```python
from build123d import *

# Parameters (mm, degrees)
SKIZZE2_R = 0.75


with BuildPart() as part:
    # Austragung1: sweep along a path in Skizze1
    with BuildLine(Plane.XY) as austragung1_path:
        Line((0, 0), (0, 15))
        ThreePointArc((0, 15), (-0.782050775, 17.292111995), (-2.802014612, 18.62819841))
        Line((-2.802014612, 18.62819841), (-26.697985388, 24.87180159))
        ThreePointArc((-26.697985388, 24.87180159), (-29.499946504, 28.47996964), (-26.736690272, 32.11786433))
        Line((-26.736690272, 32.11786433), (-4.736690272, 38.11786433))
        ThreePointArc((-4.736690272, 38.11786433), (-4.247749316, 38.216819288), (-3.75, 38.25))
        Line((-3.75, 38.25), (10.25, 38.25))
    # Skizze2 → Austragung1 (sweep)
    with BuildSketch(Plane(origin=(0, 0, 0), x_dir=(1, 0, 0), z_dir=(0, 1, 0))):
        Circle(SKIZZE2_R)
    sweep(path=austragung1_path.line)


solid = part.part
```
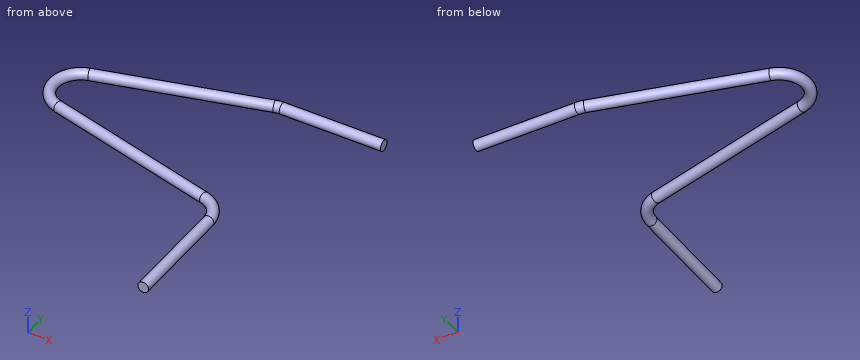
Part model, mm, in its own coordinate system. Give positions to 0.01 mm unless a question says otherwise; leave off trailing zeros. Write each loop counter-clockwise with the first axis right and the second up, starting at its lowest first coordinate (ties: lowest second). Pieces come first, ordered by that corner, then holes. Notation, with made-up numbers: M 53.5,58.5 L 83.5,58.5 A9 cw 83.5,70.5 Z; hole C -29,8.5 d7. An arc over 180 degrees is marked long. Use CSV: the item, a comma, the result in double quotes.
Item 1: Pin check, flat tip, straight feed: P1, Ø1.5, axis at x = -18, y = 31.5, coming from the -Z side (3 decimals). Stop position of the tip, or through.
Taken from the geometry:
P1,"passes through"
Item 2: Drill centre lines: probe 1 along Y at (x, z) = (-6, -0.05); probe 2 along Y at (x, z) = (-1, 0); probe 3 along X at (y, z) = (9.5, -0.35). Where is each one in solid material? Low to high.
Taken from the geometry:
probe 1,"y = 18.69 to 20.24, 37 to 38.55"
probe 2,"y = 16.2 to 18.56, 37.5 to 39"
probe 3,"x = -0.66 to 0.66"
Item 3: Slice it at A-A on z = 0. Write the cut outline in (x, y), plus the area to 3 significant figures.
Taken from the geometry:
outline,"M -26.93,32.84 A4.5 ccw -26.89,24.15 L -2.99,17.9 A3 cw -0.75,15 L -0.75,0 L 0.75,0 L 0.75,15 A4.5 ccw -2.61,19.35 L -26.51,25.6 A3 cw -26.54,31.39 L -4.54,37.39 A3 cw -3.75,37.5 L 10.25,37.5 L 10.25,39 L -3.75,39 A4.5 ccw -4.93,38.84 Z"
area,"138 mm²"
Item 4: Slice it at B-B on y = 9. Write the cut outline in (x, z), plus the area to 3 significant figures.
Taken from the geometry:
outline,"C 0,0 d1.5"
area,"1.77 mm²"
